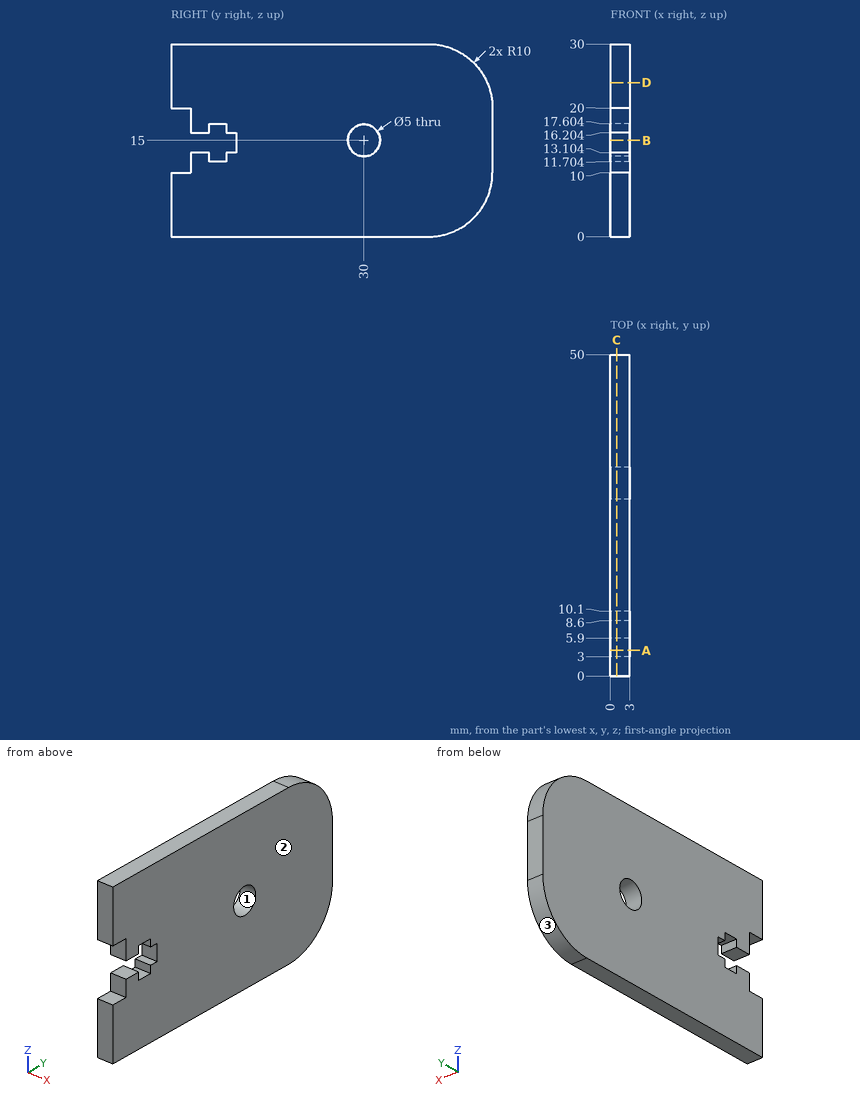
For this review, use the dimensioned drawing (mm, ordinates from the lowest corner) and the shaded views. Give positions to 0.01 mm unless a question says otherwise; leave off trailing zeros. Order: outer loops, then holes, each group sorted by start corner. A loop starts at its lowest first (then second) coordinate and runs counter-clockwise, first axis right, second up. Notation, with made-up numbers: (-36.75, 45.25) - (-11.75, 45.25) arc R21 cw to (-11.75, 55.25) - close; hole circle Ø7 at (-30.75, 39). An arc over 180 degrees is marked (long way). Use CSV: the item, a comma, the result in double quotes. Start each with the question number.
Q1. Take a section at A-A (y = 4). State the section outline as (x, z) points, and give its area (3 significant figures).
Q2. Take a section at D-D (z = 24). State the section outline as (x, y) points (1 decimal), and give its area (4 significant figures).
Q3. For P1, Ø1.5, axis at x = 1, z = 15.5, coming from the -Y side; P2, Ø4, axis at y = 30, z = 15, coming from the +X side, all flat-tipped, find the tip position at first contact; note any pin that passes through.
Q4. Draft analysis for pull direction Z (two halves, no side actions). For the marked faces 1, 2 and 3, state which applies: pulls with the +Z half, pulls with the -Z half, needs draft (parallel to the pull), parting line crosses it, or undercut.
Q5. Take a section at C-C (x = 0.95). State the section outline as (y, z) points, and give its area (3 significant figures).
Q6. For line 1 (Z direction, x = 2.4, y = 30); line 2 (Y direction, x = 0.6, z = 15); line 3 (Y direction, x = 0.25, z = 18.5), list the stretches that pass through material, from the lowest coordinate up.
Q7. Take a section at B-B (z = 15). State the section outline as (x, y) points, and give its area (3 significant figures).
Calculated:
1,outline,"(0, 0) - (3, 0) - (3, 13.1) - (0, 13.1) - close; (0, 16.2) - (3, 16.2) - (3, 30) - (0, 30) - close"
1,area,"80.7 mm²"
2,outline,"(0, 0) - (3, 0) - (3, 49.2) - (0, 49.2) - close"
2,area,"147.5 mm²"
3,P1,"stops at y = 3"
3,P2,"passes through"
4,face 1,"undercut"
4,face 2,"needs draft"
4,face 3,"pulls with the -Z half"
5,outline,"(0, 0) - (40, 0) arc R10 ccw to (50, 10) - (50, 20) arc R10 ccw to (40, 30) - (0, 30) - (0, 20) - (3, 20) - (3, 16.2) - (5.9, 16.2) - (5.9, 17.6) - (8.6, 17.6) - (8.6, 16.2) - (10.1, 16.2) - (10.1, 13.1) - (8.6, 13.1) - (8.6, 11.7) - (5.9, 11.7) - (5.9, 13.1) - (3, 13.1) - (3, 10) - (0, 10) - close; hole circle Ø5 at (30, 15)"
5,area,"1,380 mm²"
6,line 1,"z = 0 to 12.5, 17.5 to 30"
6,line 2,"y = 10.1 to 27.5, 32.5 to 50"
6,line 3,"y = 3 to 50"
7,outline,"(0, 10.1) - (3, 10.1) - (3, 27.5) - (0, 27.5) - close; (0, 32.5) - (3, 32.5) - (3, 50) - (0, 50) - close"
7,area,"105 mm²"
